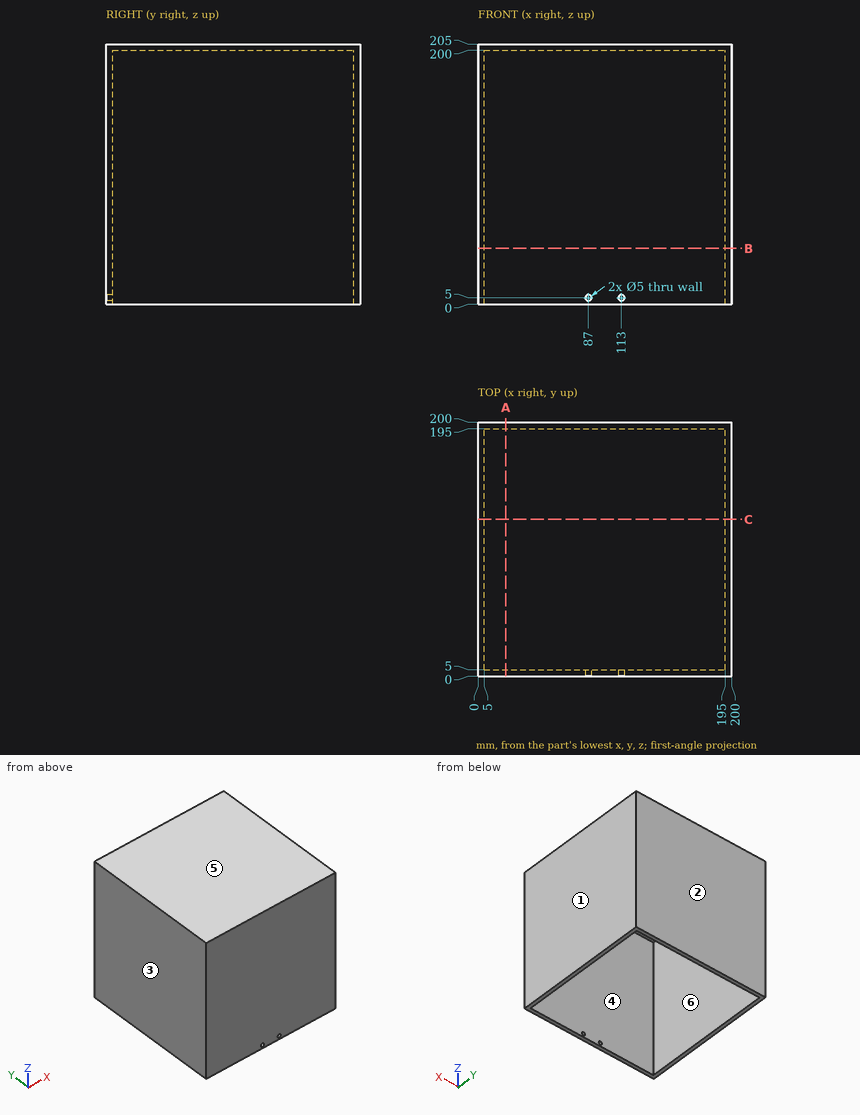
Answer from the drawing. Dimensions are ordinates in mm from the lowest x, y and z of the part. A direction names the side the tool comes from. Give positions to 0.01 mm unless a question says otherwise; leave off trailing zeros. Order: outer loops, then holes, each group sorted by start corner. A loop starts at its lowest first (then second) coordinate and runs counter-clockwise, first axis right, second up.
Item 1: For a pull along X with two mould halves and no side action, classify the marked faces 1, 2, 3 and 4 as pulls with the +X half, pulls with the -X half, needs draft (parallel to the pull), parting line crosses it, or undercut.
From the geometry:
face 1: pulls with the +X half
face 2: needs draft
face 3: pulls with the -X half
face 4: undercut
Item 2: The part is cut by section B-B, the plane z = 44. Give the vertices of the cut face in (x, y), and give its area (3 significant figures).
From the geometry:
outline: (0, 0) - (200, 0) - (200, 200) - (0, 200) - close; hole (5, 5) - (195, 5) - (195, 195) - (5, 195) - close
area: 3,900 mm2
Item 3: Given pin 1 Ø4.5 at (x, z) = (113, 5) entering from -Y; pin 2 Ø10 at (x, y) = (120, 66) entering from -Z, each flat-ended and moving along its own axis, determine where each tip first touches the part or whether it passes through.
From the geometry:
pin 1: stops at y = 195
pin 2: stops at z = 200
Item 4: The part is cut by section A-A, the plane x = 22. Give the vertices of the cut face in (y, z), and give its area (3 significant figures).
From the geometry:
outline: (0, 0) - (5, 0) - (5, 200) - (195, 200) - (195, 0) - (200, 0) - (200, 205) - (0, 205) - close
area: 3,000 mm2
Item 5: Which of the six approach directions +Z, -Z, +X, -X, +Y, -Y give full straight-line access (tool end or side, diameter ignored) to the marked faces 5 and 6?
From the geometry:
face 5: +Z, +X, -X, +Y, -Y
face 6: -Z
Item 6: Find the intervals of material crossed by probe 1 along Y at (x, z) = (96.5, 79); probe 2 along Z at (x, y) = (87, 4.05), in increasing order.
From the geometry:
probe 1: y = 0 to 5, 195 to 200
probe 2: z = 0 to 2.5, 7.5 to 205
